Check sheet for the modelled part. Datum: model origin and axes. Units: mm. Face numbers are marked on the shaded views. Coordinates: 2 decimals unless noted, no trailing zeros. Loops run counter-clockwise (first coordinate to the right, second up) from the corner with the lowest first, then second, coordinate; pieces in that order, holes last.
```python
from build123d import *

# Parameters (mm, degrees)
F0_R     = 206.375
F0_R_2   = 203.2
F1_DEPTH = 152.4
F2_R     = 206.168646
F3_DEPTH = 6.35
F4_R     = 7.62
F5_DEPTH = 25.4


with BuildPart() as f1:
    # F0 (on Top) → F1 (new body)
    with BuildSketch(Plane.XY):
        Circle(F0_R)
        Circle(F0_R_2, mode=Mode.SUBTRACT)
    extrude(amount=F1_DEPTH)

    # F2 (on Top) → F3 (join)
    with BuildSketch(Plane.XY):
        Circle(F2_R)
    extrude(amount=-F3_DEPTH)

    # F4 (on face) → F5 (cut)
    with BuildSketch(Plane.XY):
        Circle(F4_R)
    extrude(amount=-F5_DEPTH, mode=Mode.SUBTRACT)


solid = f1.part
```
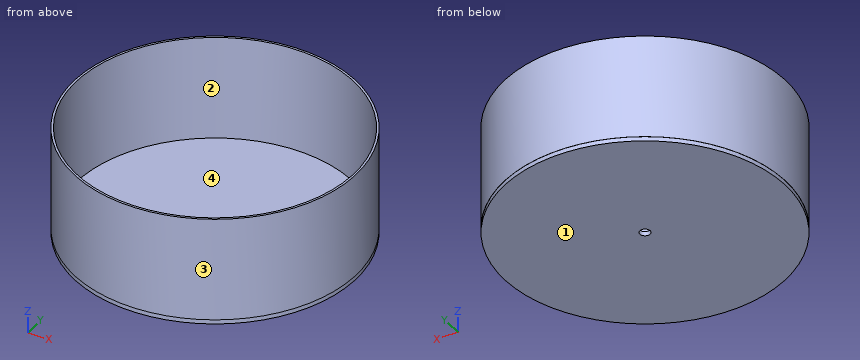
1) Depth check by flat-ended pin: pin 1 (8 mm diameter, centred on x = -85, z = 50, fed in from +Y); pin 2 (3 mm diameter, centred on y = -109.5, z = 87.5, fed in from +X); pin 3 (3 mm diameter, centred on x = 49.5, z = 130, fed in from +Y); pin 4 (13.5 mm diameter, centred on x = 0, y = 0, fed in from -Z). Enter the tip coordinate at first touch or a pass-through.
Answer sheet:
pin 1: stops at y = 189.81
pin 2: stops at x = 175.86
pin 3: stops at y = 200.72
pin 4: passes through
2) Section check A-A on x = 0. Enter the section's corners in (y, z) (3 decimals).
Answer sheet:
outline: (-206.375, 0) - (-206.169, 0) - (-206.169, -6.35) - (-7.62, -6.35) - (-7.62, 0) - (-203.2, 0) - (-203.2, 152.4) - (-206.375, 152.4) - close; (7.62, -6.35) - (206.169, -6.35) - (206.169, 0) - (206.375, 0) - (206.375, 152.4) - (203.2, 152.4) - (203.2, 0) - (7.62, 0) - close
3) Mould release check, pull along Y, two halves, no side actions. Record for the marked faces 1, 2, 3 and 4: +Y half, -Y half, draft (parallel to the pull), parting line (faces both ways), or undercut.
Answer sheet:
face 1: draft
face 2: undercut
face 3: parting line
face 4: undercut
4) Section check C-C on z = 69. Enter the section's corners in (x, y) (3 decimals), plus the area to 3 significant figures.
Answer sheet:
outline: circle Ø412.75 at (0, 0); hole circle Ø406.4 at (0, 0)
area: 4,090 mm2
5) Section check D-D on x = 111.5. Enter the section's corners in (y, z).
Answer sheet:
outline: (-173.66, 0) - (-173.42, 0) - (-173.42, -6.35) - (173.42, -6.35) - (173.42, 0) - (173.66, 0) - (173.66, 152.4) - (169.88, 152.4) - (169.88, 0) - (-169.88, 0) - (-169.88, 152.4) - (-173.66, 152.4) - close
6) Scan lines: line 1 (Y direction, x = 0, z = -3); line 2 (Z direction, x = -27, y = -156); line 3 (Y direction, x = 0, z = 95.5) (3 decimals). Record each from-to range of solid material in increasing order.
Answer sheet:
line 1: y = -206.17 to -7.62, 7.62 to 206.17
line 2: z = -6.35 to 0
line 3: y = -206.375 to -203.2, 203.2 to 206.375
